from build123d import *

# Parameters (mm, degrees)
F2_R     = 7.5
F2_R_2   = 5.5
F3_DEPTH = 3
F4_DEPTH = 5
F5_DEPTH = 5
F2_R_3   = 4.9
F6_DEPTH = 6
F7_DEPTH = 12.5


# Not quite as in the source:
# - a feature names something its author has since deleted; it is built from what else it names


with BuildPart() as f3:
    # F2 (on Top) → F3 (new body)
    with BuildSketch(Plane.XY):
        with BuildLine():
            Line((140, 9.5), (20, 9.5))
            ThreePointArc((20, 9.5), (10.5, 0), (20, -9.5))
            Line((20, -9.5), (140, -9.5))
            ThreePointArc((140, -9.5), (146.7175144213, -6.7175144213), (149.5, 0))
            ThreePointArc((149.5, 0), (146.7175144213, 6.7175144213), (140, 9.5))
        make_face()
        with Locations((20, 0)):
            Circle(F2_R, mode=Mode.SUBTRACT)
        with Locations((40, 0)):
            Circle(F2_R, mode=Mode.SUBTRACT)
        with Locations((60, 0)):
            Circle(F2_R, mode=Mode.SUBTRACT)
        with Locations((80, 0)):
            Circle(F2_R, mode=Mode.SUBTRACT)
        with Locations((100, 0)):
            Circle(F2_R, mode=Mode.SUBTRACT)
        with Locations((120, 0)):
            Circle(F2_R, mode=Mode.SUBTRACT)
        with Locations((140, 0)):
            Circle(F2_R, mode=Mode.SUBTRACT)
        with Locations((20, 0)):
            Circle(F2_R)
        with Locations((20, 0)):
            Circle(F2_R_2, mode=Mode.SUBTRACT)
        with Locations((40, 0)):
            Circle(F2_R)
        with Locations((40, 0)):
            Circle(F2_R_2, mode=Mode.SUBTRACT)
        with Locations((60, 0)):
            Circle(F2_R)
        with Locations((60, 0)):
            Circle(F2_R_2, mode=Mode.SUBTRACT)
        with Locations((80, 0)):
            Circle(F2_R)
        with Locations((80, 0)):
            Circle(F2_R_2, mode=Mode.SUBTRACT)
        with Locations((100, 0)):
            Circle(F2_R)
        with Locations((100, 0)):
            Circle(F2_R_2, mode=Mode.SUBTRACT)
        with Locations((120, 0)):
            Circle(F2_R)
        with Locations((120, 0)):
            Circle(F2_R_2, mode=Mode.SUBTRACT)
        with Locations((140, 0)):
            Circle(F2_R)
        with Locations((140, 0)):
            Circle(F2_R_2, mode=Mode.SUBTRACT)
    extrude(amount=F3_DEPTH)

    # F2 (on Top) → F4 (join)
    with BuildSketch(Plane.XY):
        with Locations((20, 0)):
            Circle(F2_R)
        with Locations((20, 0)):
            Circle(F2_R_2, mode=Mode.SUBTRACT)
        with Locations((40, 0)):
            Circle(F2_R)
        with Locations((40, 0)):
            Circle(F2_R_2, mode=Mode.SUBTRACT)
        with Locations((60, 0)):
            Circle(F2_R)
        with Locations((60, 0)):
            Circle(F2_R_2, mode=Mode.SUBTRACT)
        with Locations((80, 0)):
            Circle(F2_R)
        with Locations((80, 0)):
            Circle(F2_R_2, mode=Mode.SUBTRACT)
        with Locations((100, 0)):
            Circle(F2_R)
        with Locations((100, 0)):
            Circle(F2_R_2, mode=Mode.SUBTRACT)
        with Locations((120, 0)):
            Circle(F2_R)
        with Locations((120, 0)):
            Circle(F2_R_2, mode=Mode.SUBTRACT)
        with Locations((140, 0)):
            Circle(F2_R)
        with Locations((140, 0)):
            Circle(F2_R_2, mode=Mode.SUBTRACT)
    extrude(amount=F4_DEPTH)

    # F2 (on Top) → F5 (join)
    with BuildSketch(Plane.XY):
        with Locations((140, 0)):
            Circle(F2_R)
        with Locations((140, 0)):
            Circle(F2_R_2, mode=Mode.SUBTRACT)
    extrude(amount=F5_DEPTH)

    # F2 (on Top) → F6 (join)
    with BuildSketch(Plane.XY):
        with Locations((20, 0)):
            Circle(F2_R)
        with Locations((20, 0)):
            Circle(F2_R_2, mode=Mode.SUBTRACT)
        with Locations((20, 0)):
            Circle(F2_R_2)
        with Locations((20, 0)):
            Circle(F2_R_3, mode=Mode.SUBTRACT)
    extrude(amount=F6_DEPTH)

    # F2 (on Top) → F7 (join)
    with BuildSketch(Plane.XY):
        with Locations((20, 0)):
            Circle(F2_R_3)
        with BuildLine():
            Line((22.2847319318, -2.45), (20, -2.45))
            Line((20, -2.45), (17.7152680682, -2.45))
            ThreePointArc((17.7152680682, -2.45), (16.65, 0), (17.7152680682, 2.45))
            Line((17.7152680682, 2.45), (20, 2.45))
            Line((20, 2.45), (22.2847319318, 2.45))
            ThreePointArc((22.2847319318, 2.45), (23.35, 0), (22.2847319318, -2.45))
        make_face(mode=Mode.SUBTRACT)
    extrude(amount=F7_DEPTH)

    # F9 (on plane+point) → F10 (revolve)
    with BuildSketch(Plane.XZ):
        Polygon((25.15, 11.75), (24.9, 12.5), (24.9, 11), align=None)
    revolve(axis=Axis((20, 0, 6.25), (0, 0, 1)))


solid = f3.part
Check sheet for the modelled part. Datum: model origin and axes. Units: mm. A direction names the side the tool comes from. Round coordinates to 2 decimals unless told otherwise and drop trailing zeros. Loops run counter-clockwise (first coordinate to the right, second up) from the corner with the lowest first, then second, coordinate; pieces in that order, holes last. Notation, with made-up numbers: (14.25, 87) -> (32.25, 87) arc R31 ccw to (32.25, 112) -> close; hole circle Ø9 at (-33.5, 55.5). An arc over 180 degrees is marked (long way). Put each result on its own line as item: value. Start each with the question number.
1. Section check A-A (x = 80). Enter the section's corners in (y, z).
2. Access from +Z, -Z, +X, -X, +Y, -Y to the whole of each face (thin tool, end or side, straight path). Record for faces 1 (the face through (36, 4, 5)), 2 (the face through (16.65, -0.04, 6.16)), 3 (the face through (127.154, 2.253, 3.986)).
3. Scan lines: probe 1 along Y at (x, z) = (80, 3.5); probe 2 along Y at (x, z) = (100, 2.2); probe 3 along Z at (x, y) = (118, -8). Record each from-to range of solid material in increasing order.
4. Gauge pin test, flat ends, axial feed: pin 1 (7.5 mm diameter, centred on x = 77, y = -0.5, fed in from +Z); pin 2 (1.5 mm diameter, centred on y = 1.5, z = 5, fed in from +X); pin 3 (1.4 mm diameter, centred on x = 20.5, z = 6.5, fed in from +Y). Record the tip position at first contact, or that the pin passes through.
5. Draft check along X on faces 4 (the face through (134.505, 0.242, 2.465)), 5 (the face through (16.11, -2.98, 8.46)), 6 (the face through (96, 4, 5)). Enter one of: +X half, -X half, draft (parallel to the pull), parting line (faces both ways), or undercut.
6. Section check B-B (x = 43). Enter the section's corners in (y, z), plus the area to 3 significant figures.
Findings:
1. outline: (-9.5, 0) -> (-5.5, 0) -> (-5.5, 5) -> (-7.5, 5) -> (-7.5, 3) -> (-9.5, 3) -> close; (5.5, 0) -> (9.5, 0) -> (9.5, 3) -> (7.5, 3) -> (7.5, 5) -> (5.5, 5) -> close
2. face 1: +Z, +X, +Y, -Y
2. face 2: +Z, -Z
2. face 3: +Z
3. probe 1: y = -7.5 to -5.5, 5.5 to 7.5
3. probe 2: y = -9.5 to -5.5, 5.5 to 9.5
3. probe 3: z = 0 to 3
4. pin 1: stops at z = 5
4. pin 2: stops at x = 147.46
4. pin 3: stops at y = 7.5
5. face 4: undercut
5. face 5: parting line
5. face 6: draft
6. outline: (-9.5, 0) -> (-4.61, 0) -> (-4.61, 5) -> (-6.87, 5) -> (-6.87, 3) -> (-9.5, 3) -> close; (4.61, 0) -> (9.5, 0) -> (9.5, 3) -> (6.87, 3) -> (6.87, 5) -> (4.61, 5) -> close
6. area: 38.4 mm^2
